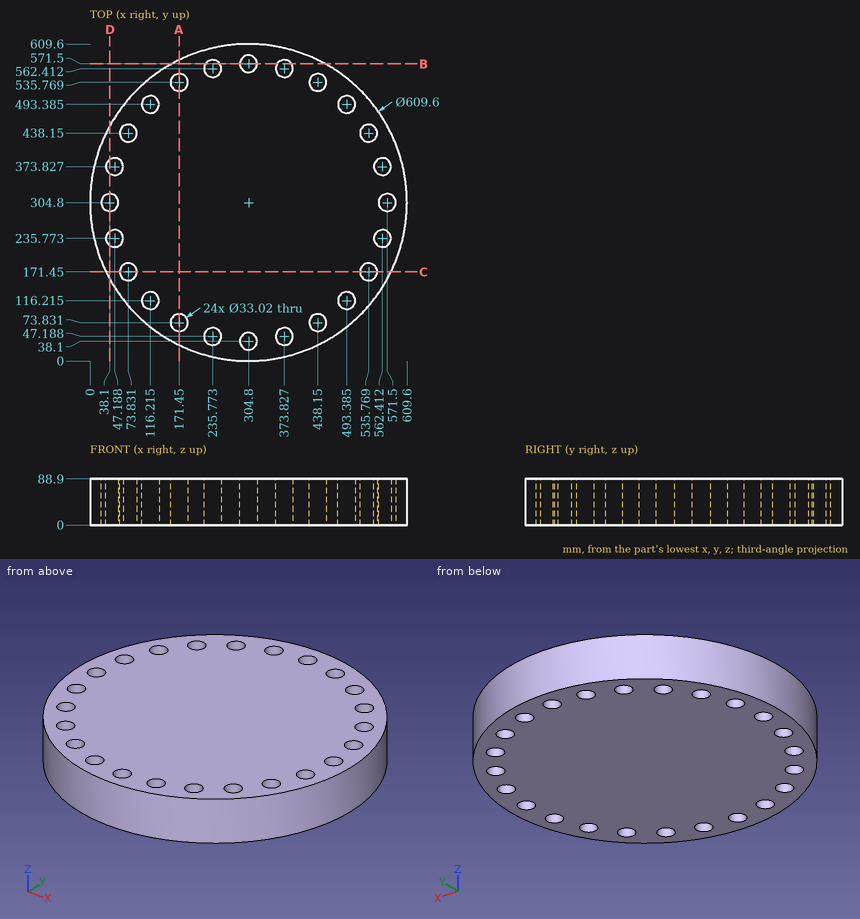
Answer from the drawing. Dimensions are ordinates in mm from the lowest x, y and z of the part. Coordinates: 2 decimals unless noted, no trailing zeros. Order: outer loops, then holes, each group sorted by start corner. A loop starts at its lowest first (then second) coordinate and runs counter-clockwise, first axis right, second up. Notation, with made-up numbers: (89.5, -8.75) - (98.5, -8.75) arc R25 ccw to (98.5, 10.25) - close; hole circle Ø3 at (89, 8). An arc over 180 degrees is marked (long way). Put each result on its own line as item: value. Start each with the question number.
1) Find section A-A (x = 171.45). Give the vertices of the cut face in (y, z).
2) Flat-ended cylindrical pins translate along their axes: pin 1 (5 mm diameter, centred on x = 232, z = 62.5, fed in from -Y); pin 2 (5 mm diameter, centred on y = 267, z = 39.5, fed in from -X); pin 3 (2 mm diameter, centred on x = 422.5, z = 66, fed in from +Y) (1 decimal). Find the tip coordinate at first contact, or state that the pin passes through.
3) Find the intervals of material crossed by line 1 (X direction, y = 167, z = 5); line 2 (X direction, y = 563, z = 14) (1 decimal); line 3 (Y direction, x = 538, z = 16) (1 decimal), in increasing order. Write a range as from..to.
4) Find section B-B (y = 571.5). Give the vertices of the cut face in (x, z).
Results list:
1. outline: (30.72, 0) - (57.32, 0) - (57.32, 88.9) - (30.72, 88.9) - close; (90.34, 0) - (519.26, 0) - (519.26, 88.9) - (90.34, 88.9) - close; (552.28, 0) - (578.88, 0) - (578.88, 88.9) - (552.28, 88.9) - close
2. pin 1: stops at y = 8.22
2. pin 2: stops at x = 2.05
2. pin 3: stops at y = 586.4
3. line 1: x = 32.93..57.93, 89.73..519.87, 551.67..576.67
3. line 2: x = 142.8..219.3, 252.3..290.6, 319..357.3, 390.3..466.8
3. line 3: y = 108.5..155.1, 187.8..421.8, 454.5..501.1
4. outline: (157.24, 0) - (221.99, 0) - (221.99, 88.9) - (157.24, 88.9) - close; (249.56, 0) - (288.29, 0) - (288.29, 88.9) - (249.56, 88.9) - close; (321.31, 0) - (360.04, 0) - (360.04, 88.9) - (321.31, 88.9) - close; (387.61, 0) - (452.36, 0) - (452.36, 88.9) - (387.61, 88.9) - close
